Read the model definition and answer for the solid it produces. Units are mm, in the model's axes. A direction names the side the tool comes from. Give positions to 0.01 mm unless a question says otherwise; leave off trailing zeros. Order: outer loops, then holes, each group sorted by start corner. A loop starts at its lowest first (then second) coordinate and runs counter-clockwise, first axis right, second up.
```python
from build123d import *

# Parameters (mm, degrees)
BOSS_EXTRUDE1_DEPTH = 5
SKETCH4_R           = 15.811388301
BOSS_EXTRUDE2_DEPTH = 15


with BuildPart() as part:
    # Sketch1 → Boss-Extrude1 (new, symmetric)
    with BuildSketch(Plane.XY):
        with BuildLine():
            Line((-15, -75), (-15, 75))
            Line((-15, 75), (15, 75))
            Line((15, 75), (15, -75))
            ThreePointArc((15, -75), (0, -90), (-15, -75))
        make_face()
    extrude(amount=BOSS_EXTRUDE1_DEPTH, both=True)

    # Sketch4 → Boss-Extrude2 (add)
    with BuildSketch(Plane(origin=(0, 75, 0), x_dir=(1, 0, 0), z_dir=(0, 1, 0))):
        with Locations(Location((0, 0, 0), (0, 0, 270))):
            Circle(SKETCH4_R)
    extrude(amount=-BOSS_EXTRUDE2_DEPTH)

    # Sketch6 → Cut-Revolve3 (revolve, cut)
    with BuildSketch(Plane.XY):
        with BuildLine():
            Line((0, 75), (10, 75))
            ThreePointArc((10, 75), (7.071067812, 67.928932188), (0, 65))
            Line((0, 65), (0, 75))
        make_face()
    revolve(axis=Axis((0, 75, 0), (0, -1, 0)), mode=Mode.SUBTRACT)


solid = part.part
```
1) For a pull along Z with two mould halves and no side action, classify faces 4 (the face through (0, 60, -9)), 5 (the face through (-9.62, 67.6, -12.55)), 6 (the face through (0, -14, -5)) as released by +Z, released by -Z, zero draft, split by the parting line, or undercut.
Final values:
face 4: zero draft
face 5: split by the parting line
face 6: released by -Z
2) The part is cut by section A-A on x = 0. Determine the outline of the cut face in (y, z).
Final values:
outline: (-90, -5) - (60, -5) - (60, -15.81) - (75, -15.81) - (75, -10) arc R10 cw to (75, 10) - (75, 15.81) - (60, 15.81) - (60, 5) - (-90, 5) - close
3) Given pin 1 (3 mm diameter, centred on x = 2, z = -8.5, fed in from +Y); pin 2 (2 mm diameter, centred on x = 3, y = -6, fed in from -Z); pin 3 (11 mm diameter, centred on y = -1, z = 2, fed in from -X); pin 4 (3 mm diameter, centred on x = 1, z = 11, fed in from -Y), each flat-ended and moving along its own axis, determine where each tip first touches the part or whether it passes through.
Final values:
pin 1: stops at y = 75
pin 2: stops at z = -5
pin 3: stops at x = -15
pin 4: stops at y = 60
4) A tool of negligible diameter and unlimited length cuts with its end or side. For faces 1 (the face through (0, -14, 5)), 2 (the face through (-15, -8, 0)), 3 (the face through (15, -7, 0)), from which of +Z, -Z, +X, -X, +Y, -Y can it reach the whole face along a straight path? Write none if from no direction.
Final values:
face 1: +Z, +X, -X, -Y
face 2: +Z, -Z, -X, -Y
face 3: +Z, -Z, +X, -Y
5) The part is cut by section C-C on y = 12.5. Determine the outline of the cut face in (x, z).
Final values:
outline: (-15, -5) - (15, -5) - (15, 5) - (-15, 5) - close
6) The part is cut by section D-D on x = 6.5. Determine the outline of the cut face in (y, z).
Final values:
outline: (-88.52, -5) - (60, -5) - (60, -14.41) - (75, -14.41) - (75, -7.6) arc R7.6 cw to (75, 7.6) - (75, 14.41) - (60, 14.41) - (60, 5) - (-88.52, 5) - close
7) The part is cut by section B-B on z = 0. Determine the outline of the cut face in (x, y), and give its area (3 significant figures).
Final values:
outline: (-15.81, 60) - (-15, 60) - (-15, -75) arc R15 ccw to (15, -75) - (15, 60) - (15.81, 60) - (15.81, 75) - (10, 75) arc R10 cw to (-10, 75) - (-15.81, 75) - close
area: 4,720 mm2
8) Consider L1, parallel to Y at x = 6, z = 13; L2, parallel to Z at x = 9, y = -73; L3, parallel to X at y = -20, z = 2.5. Determine where each line is inside the solid, lowest interval first.
Final values:
L1: y = 60 to 75
L2: z = -5 to 5
L3: x = -15 to 15
